Check sheet for the modelled part. Datum: model origin and axes. Units: mm. Face numbers are marked on the shaded views. A direction names the side the tool comes from. Coordinates: 2 decimals unless noted, no trailing zeros. Loops run counter-clockwise (first coordinate to the right, second up) from the corner with the lowest first, then second, coordinate; pieces in that order, holes last. Notation, with made-up numbers: M -16.75,65.25 L 11.25,65.25 A27 cw 11.25,99.25 Z; hole C 9.25,-30.75 d1. An arc over 180 degrees is marked long. Return JSON: item names as keys, results as strings.
from build123d import *

# Parameters (mm, degrees)
BOSS_EXTRUDE1_DEPTH = 7
BOSS_EXTRUDE2_DEPTH = 8
BOSS_EXTRUDE3_DEPTH = 12
CUT_EXTRUDE1_REACH  = 52.149
SKETCH4_R           = 50
SKETCH4_R_2         = 36.5


with BuildPart() as part:
    # Sketch1 → Boss-Extrude1 (new body)
    with BuildSketch(Plane(origin=(0, 0, 0), x_dir=(1, 0, 0), z_dir=(0, 1, 0))):
        with BuildLine():
            Line((0, 11), (34.803017111, 11))
            ThreePointArc((34.803017111, 11), (36.5, 0), (34.803017111, -11))
            Line((34.803017111, -11), (0, -11))
            ThreePointArc((0, -11), (11, 0), (0, 11))
        make_face()
    extrude(amount=BOSS_EXTRUDE1_DEPTH)

    # Sketch2 → Boss-Extrude2 (add)
    with BuildSketch(Plane(origin=(0, 7, 0), x_dir=(1, 0, 0), z_dir=(0, 1, 0))):
        with BuildLine():
            Line((3.666174209, 6.35), (35.943392995, 6.35))
            ThreePointArc((35.943392995, 6.35), (36.5, 0), (35.943392995, -6.35))
            Line((35.943392995, -6.35), (3.666174209, -6.35))
            Line((3.666174209, -6.35), (7.332348419, 0))
            Line((7.332348419, 0), (3.666174209, 6.35))
        make_face()
    extrude(amount=BOSS_EXTRUDE2_DEPTH)

    # Sketch3 → Boss-Extrude3 (add)
    with BuildSketch(Plane(origin=(26.6, 0, 0), x_dir=(0, 0, -1), z_dir=(1, 0, 0))):
        with BuildLine():
            Line((-15, -1), (15, -1))
            ThreePointArc((15, -1), (25, 9), (15, 19))
            Line((15, 19), (-15, 19))
            ThreePointArc((-15, 19), (-25, 9), (-15, -1))
        make_face()
    extrude(amount=BOSS_EXTRUDE3_DEPTH)

    # Sketch4 → Cut-Extrude1 (cut, up to next)
    with BuildSketch(Plane(origin=(0, 19, 0), x_dir=(1, 0, 0), z_dir=(0, 1, 0)), mode=Mode.PRIVATE) as cut_extrude1_sk1:
        Circle(SKETCH4_R)
        Circle(SKETCH4_R_2, mode=Mode.SUBTRACT)
    cut_extrude1_tool1 = extrude(cut_extrude1_sk1.sketch, amount=-CUT_EXTRUDE1_REACH, mode=Mode.PRIVATE) & part.part
    add(cut_extrude1_tool1.solids().sort_by_distance((-48.585786, 19, 0))[0], mode=Mode.SUBTRACT)


solid = part.part
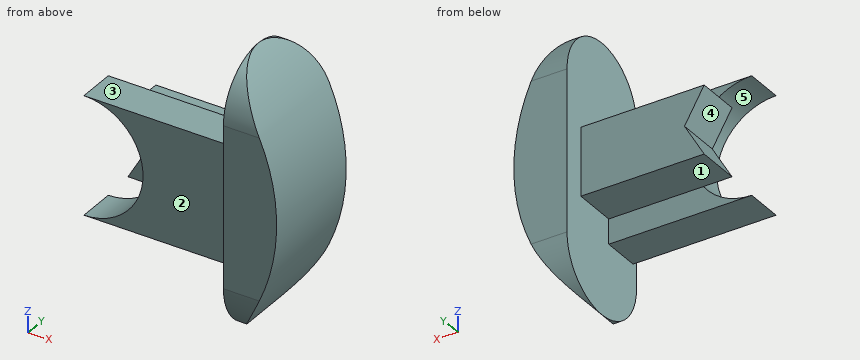
1) Section check D-D on z = 4.5. Record the cut outline in (x, y), then the cut area to 3 significant figures.
Answers:
{"outline": "M 4.73,7 L 10.04,7 L 10.04,0 L 26.6,0 L 26.6,-1 L 36.22,-1 L 36.22,19 L 26.6,19 L 26.6,15 L 4.73,15 Z", "area": "483 mm²"}
2) Go/stop test with flat-tipped pins: pin 1 Ø8 at (y, z) = (12.5, 4) entering from +X; pin 2 Ø3.5 at (x, z) = (9, -2.5) entering from -Y; pin 3 Ø3 at (x, y) = (23, 1) entering from +Z. Record where each tip stops, or that it passes through.
Answers:
{"pin 1": "x = 36.5", "pin 2": "y = 0", "pin 3": "z = 11"}
3) Scan lines: line 1 along Y through (x, z) = (8.5, 5.5); line 2 along Z through (x, y) = (13, 5.25); line 3 along Z through (x, y) = (23, 14). Record each from-to range of solid material in increasing order. Write a range as [from, to].
Answers:
{"line 1": "[7, 15]", "line 2": "[-11, 11]", "line 3": "[-6.35, 6.35]"}
4) Section check B-B on z = -1. Record the cut outline in (x, y) (3 decimals).
Answers:
{"outline": "M 6.755,7 L 10.954,7 L 10.954,0 L 26.6,0 L 26.6,-1 L 36.486,-1 L 36.486,19 L 26.6,19 L 26.6,15 L 6.755,15 Z"}
5) Set-up check for the marked faces 1, 2, 3, 4 and 5: record each of +Z, -Z, +X, -X, +Y, -Y from which the full face is reachable in a straight line by a thin tool's end or side.
Answers:
{"face 1": "-Z, -X, +Y", "face 2": "+Z, -Z, -X, -Y", "face 3": "+Z, -X, +Y, -Y", "face 4": "-X, +Y, -Y", "face 5": "-X, -Y"}
6) Section check A-A on x = 18.5. Record the cut outline in (y, z), then the cut area to 3 significant figures.
Answers:
{"outline": "M 0,-11 L 7,-11 L 7,-6.35 L 15,-6.35 L 15,6.35 L 7,6.35 L 7,11 L 0,11 Z", "area": "256 mm²"}
7) Section check C-C on y = 1. Record the cut outline in (x, z).
Answers:
{"outline": "M 0,-11 L 26.6,-11 L 26.6,-21 L 29.85,-21 A36.5 ccw 29.85,21 L 26.6,21 L 26.6,11 L 0,11 A11 cw Z"}
